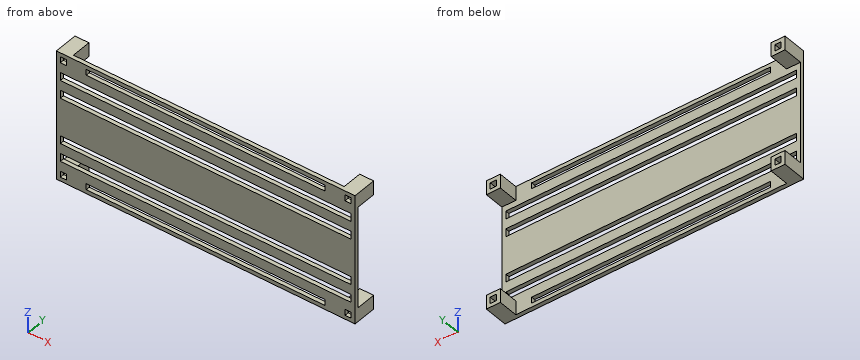
```python
from build123d import *

# Parameters (mm, degrees)
SKETCH1_W               = 150
SKETCH1_H               = 65
BOSS_EXTRUDE1_DEPTH     = 2
BOSS_EXTRUDE2_START     = 2
SKETCH2_W               = 3
SKETCH2_H               = 3
BOSS_EXTRUDE2_DEPTH     = 50
CUT_EXTRUDE2_DEPTH      = 96.818839484
CUT_EXTRUDE2_DEPTH_BACK = 96.818839484
SKETCH4_W               = 120
SKETCH4_H               = 3
SKETCH4_W_2             = 146
SKETCH4_H_2             = 4
SKETCH5_W               = 7
SKETCH5_H               = 7
SKETCH5_W_2             = 3.2
SKETCH5_H_2             = 3.2
BOSS_EXTRUDE3_DEPTH     = 50
SKETCH2_3_W             = 3
SKETCH2_3_H             = 3
CUT_EXTRUDE3_DEPTH      = 52
CUT_EXTRUDE4_DEPTH      = 97.877499968
CUT_EXTRUDE4_DEPTH_BACK = 97.877499968
SKETCH6_W               = 182.778356439
SKETCH6_H               = 52.909524232


with BuildPart() as part:
    # Sketch1 → Boss-Extrude1 (new body)
    with BuildSketch(Plane(origin=(0, 0, 0), x_dir=(1, 0, 0), z_dir=(0, 1, 0))):
        Rectangle(SKETCH1_W, SKETCH1_H)
    extrude(amount=BOSS_EXTRUDE1_DEPTH)

    # Sketch2 → Boss-Extrude2 (add)
    with BuildSketch(Plane(origin=(0, 0, 0), x_dir=(1, 0, 0), z_dir=(0, 1, 0)).offset(BOSS_EXTRUDE2_START)):
        with Locations((71.5, 29)):
            Rectangle(SKETCH2_W, SKETCH2_H)
        with Locations((-71.5, 29)):
            Rectangle(SKETCH2_W, SKETCH2_H)
        with Locations((-71.5, -29)):
            Rectangle(SKETCH2_W, SKETCH2_H)
        with Locations((71.5, -29)):
            Rectangle(SKETCH2_W, SKETCH2_H)
    extrude(amount=BOSS_EXTRUDE2_DEPTH)

    # Sketch4 → Cut-Extrude2 (cut, two sides: drawn at the far end of the back side and taken through both)
    with BuildSketch(Plane(origin=(0, 2, 0), x_dir=(1, 0, 0), z_dir=(0, 1, 0)).offset(-CUT_EXTRUDE2_DEPTH_BACK)):
        with Locations((0, 29)):
            Rectangle(SKETCH4_W, SKETCH4_H)
        with Locations((0, 20.5)):
            Rectangle(SKETCH4_W_2, SKETCH4_H_2)
        with Locations((0, 11.5)):
            Rectangle(SKETCH4_W_2, SKETCH4_H_2)
        with Locations((0, -11.5)):
            Rectangle(SKETCH4_W_2, SKETCH4_H_2)
        with Locations((0, -20.5)):
            Rectangle(SKETCH4_W_2, SKETCH4_H_2)
        with Locations((0, -29)):
            Rectangle(SKETCH4_W, SKETCH4_H)
    extrude(amount=CUT_EXTRUDE2_DEPTH + CUT_EXTRUDE2_DEPTH_BACK, mode=Mode.SUBTRACT)

    # Sketch5 → Boss-Extrude3 (add)
    # profile 1 of 4: a face of its own
    with BuildSketch(Plane(origin=(0, 2, 0), x_dir=(1, 0, 0), z_dir=(0, 1, 0))):
        with Locations((71.5, 29)):
            Rectangle(SKETCH5_W, SKETCH5_H)
        with Locations((71.5, 29)):
            Rectangle(SKETCH5_W_2, SKETCH5_H_2, mode=Mode.SUBTRACT)
    # profile 2 of 4: a face of its own
    with BuildSketch(Plane(origin=(0, 2, 0), x_dir=(1, 0, 0), z_dir=(0, 1, 0))):
        with Locations((71.5, -29)):
            Rectangle(SKETCH5_W, SKETCH5_H)
        with Locations((71.5, -29)):
            Rectangle(SKETCH5_W_2, SKETCH5_H_2, mode=Mode.SUBTRACT)
    # profile 3 of 4: a face of its own
    with BuildSketch(Plane(origin=(0, 2, 0), x_dir=(1, 0, 0), z_dir=(0, 1, 0))):
        with Locations((-71.5, -29)):
            Rectangle(SKETCH5_W, SKETCH5_H)
        with Locations((-71.5, -29)):
            Rectangle(SKETCH5_W_2, SKETCH5_H_2, mode=Mode.SUBTRACT)
    # profile 4 of 4: a face of its own
    with BuildSketch(Plane(origin=(0, 2, 0), x_dir=(1, 0, 0), z_dir=(0, 1, 0))):
        with Locations((-71.5, 29)):
            Rectangle(SKETCH5_W, SKETCH5_H)
        with Locations((-71.5, 29)):
            Rectangle(SKETCH5_W_2, SKETCH5_H_2, mode=Mode.SUBTRACT)
    extrude(amount=BOSS_EXTRUDE3_DEPTH)

    # Sketch2<3> → Cut-Extrude3 (cut)
    with BuildSketch(Plane(origin=(0, 0, 0), x_dir=(1, 0, 0), z_dir=(0, 1, 0))):
        with Locations((71.5, 29)):
            Rectangle(SKETCH2_3_W, SKETCH2_3_H)
        with Locations((-71.5, 29)):
            Rectangle(SKETCH2_3_W, SKETCH2_3_H)
        with Locations((-71.5, -29)):
            Rectangle(SKETCH2_3_W, SKETCH2_3_H)
        with Locations((71.5, -29)):
            Rectangle(SKETCH2_3_W, SKETCH2_3_H)
    extrude(amount=CUT_EXTRUDE3_DEPTH, mode=Mode.SUBTRACT)

    # Sketch6 → Cut-Extrude4 (cut, two sides: drawn at the far end of the back side and taken through both)
    with BuildSketch(Plane.XY.offset(-CUT_EXTRUDE4_DEPTH_BACK)):
        with Locations((0.082930289, 38.454762116)):
            Rectangle(SKETCH6_W, SKETCH6_H)
    extrude(amount=CUT_EXTRUDE4_DEPTH + CUT_EXTRUDE4_DEPTH_BACK, mode=Mode.SUBTRACT)


solid = part.part
```
Geometry check sheet. Reference: the model listing, model coordinates, mm. Round coordinates to 2 decimals unless told otherwise and drop trailing zeros. Loops run counter-clockwise (first coordinate to the right, second up) from the corner with the lowest first, then second, coordinate; pieces in that order, holes last. Notation, with made-up numbers: (55.5, 45) -> (93.5, 45) arc R9 ccw to (93.5, 59) -> close; hole circle Ø9 at (35, 18). An arc over 180 degrees is marked (long way). Use a Markdown table: item, result.
(1) Sectioned sample at B-B (x = 46.5). Enter the section's corners in (y, z).
Calculated:
| item | result |
|---|---|
| outline | (0, -32.5) -> (2, -32.5) -> (2, -30.5) -> (0, -30.5) -> close; (0, -27.5) -> (2, -27.5) -> (2, -22.5) -> (0, -22.5) -> close; (0, -18.5) -> (2, -18.5) -> (2, -13.5) -> (0, -13.5) -> close; (0, -9.5) -> (2, -9.5) -> (2, 9.5) -> (0, 9.5) -> close; (0, 13.5) -> (2, 13.5) -> (2, 18.5) -> (0, 18.5) -> close; (0, 22.5) -> (2, 22.5) -> (2, 27.5) -> (0, 27.5) -> close; (0, 30.5) -> (2, 30.5) -> (2, 32.5) -> (0, 32.5) -> close |
(2) Scan line: probe 1 along Y at (x, z) = (-15, -14). Record every from-to range of solid material in increasing order.
Calculated:
| item | result |
|---|---|
| probe 1 | 0 to 2 |
(3) Go/stop test with a flat-tipped pin: P1, Ø10, axis at x = 10, z = -6, coming from the +Y side. Record where the tip stops, or that it passes through.
Calculated:
| item | result |
|---|---|
| P1 | y = 2 |
(4) Sectioned sample at C-C (z = 20). Enter the section's corners in (x, y).
Calculated:
| item | result |
|---|---|
| outline | (-75, 0) -> (-73, 0) -> (-73, 2) -> (-75, 2) -> close; (73, 0) -> (75, 0) -> (75, 2) -> (73, 2) -> close |
(5) Sectioned sample at A-A (y = 5.5). Give the number of separate pieces and of enclosed holes in the cut face, then the cut area to 3 significant figures.
Calculated:
| item | result |
|---|---|
| separate pieces | 4 |
| enclosed holes | 4 |
| area | 155 mm² |
(6) Sectioned sample at D-D (z = 0.5). Enter the section's corners in (x, y), then the cut area to 3 significant figures.
Calculated:
| item | result |
|---|---|
| outline | (-75, 0) -> (75, 0) -> (75, 2) -> (-75, 2) -> close |
| area | 300 mm² |
